```python
from build123d import *

# Parameters (mm, degrees)
SKETCH1_R               = 2.5
SKETCH1_W               = 6.5
SKETCH1_H               = 5
BOSS_EXTRUDE1_DEPTH     = 3
SKETCH1_3_W             = 6.5
SKETCH1_3_H             = 5
BOSS_EXTRUDE2_DEPTH     = 5.5
BOSS_EXTRUDE3_START     = -3
SKETCH2_W               = 3
SKETCH2_H               = 24
SKETCH2_H_2             = 3
SKETCH2_W_2             = 13
BOSS_EXTRUDE3_DEPTH     = 46
CUT_EXTRUDE1_DEPTH      = 56.497747702
CUT_EXTRUDE1_DEPTH_BACK = 56.497747702
CUT_EXTRUDE2_START      = -1
SKETCH4_R               = 1.75
CUT_EXTRUDE2_DEPTH      = 57.201398584
SKETCH4_2_R             = 1.75
CUT_EXTRUDE3_DEPTH      = 58.201398584
FILLET1_R               = 0.7


with BuildPart() as part:
    # Sketch1 → Boss-Extrude1 (new body)
    # profile 1 of 3: a face of its own
    with BuildSketch(Plane(origin=(0, 0, 0), x_dir=(1, 0, 0), z_dir=(0, 1, 0))):
        Polygon((-8, 30), (-8, 0), (-3.25, 0), (-3.25, 5), (3.25, 5), (3.25, 0), (8, 0), (8, 30), (3.25, 30), (3.25, 25), (-3.25, 25), (-3.25, 30), align=None)
        with Locations(Location((0, 15, 0), (0, 0, 270))):
            Circle(SKETCH1_R, mode=Mode.SUBTRACT)
    # profile 2 of 3: a face of its own
    with BuildSketch(Plane(origin=(0, 0, 0), x_dir=(1, 0, 0), z_dir=(0, 1, 0))):
        with Locations((0, 2.5)):
            Rectangle(SKETCH1_W, SKETCH1_H)
    # profile 3 of 3: a face of its own
    with BuildSketch(Plane(origin=(0, 0, 0), x_dir=(1, 0, 0), z_dir=(0, 1, 0))):
        with Locations((0, 27.5)):
            Rectangle(SKETCH1_W, SKETCH1_H)
    extrude(amount=BOSS_EXTRUDE1_DEPTH)

    # Sketch1<3> → Boss-Extrude2 (add)
    with BuildSketch(Plane(origin=(0, 0, 0), x_dir=(1, 0, 0), z_dir=(0, 1, 0))):
        with Locations((0, 27.5)):
            Rectangle(SKETCH1_3_W, SKETCH1_3_H)
        with Locations((0, 2.5)):
            Rectangle(SKETCH1_3_W, SKETCH1_3_H)
    extrude(amount=-BOSS_EXTRUDE2_DEPTH)

    # Sketch2 → Boss-Extrude3 (add)
    with BuildSketch(Plane(origin=(0, 3, 0), x_dir=(1, 0, 0), z_dir=(0, 1, 0)).offset(BOSS_EXTRUDE3_START)):
        with Locations((-6.5, 15)):
            Rectangle(SKETCH2_W, SKETCH2_H)
        with Locations((-6.5, 1.5)):
            Rectangle(SKETCH2_W, SKETCH2_H_2)
        with Locations((-6.5, 28.5)):
            Rectangle(SKETCH2_W, SKETCH2_H_2)
        with Locations((1.5, 28.5)):
            Rectangle(SKETCH2_W_2, SKETCH2_H_2)
        with Locations((1.5, 1.5)):
            Rectangle(SKETCH2_W_2, SKETCH2_H_2)
    extrude(amount=BOSS_EXTRUDE3_DEPTH)

    # Sketch3 → Cut-Extrude1 (cut, two sides: drawn at the far end of the back side and taken through both)
    with BuildSketch(Plane(origin=(0, 0, -30), x_dir=(-1, 0, 0), z_dir=(0, 0, -1)).offset(-CUT_EXTRUDE1_DEPTH_BACK)):
        Polygon((-8, 6), (2, 46), (-8, 46), align=None)
    extrude(amount=CUT_EXTRUDE1_DEPTH + CUT_EXTRUDE1_DEPTH_BACK, mode=Mode.SUBTRACT)

    # Sketch4 → Cut-Extrude2 (cut, through all)
    # profile 1 of 2: a face of its own
    with BuildSketch(Plane.ZY.offset(8).offset(CUT_EXTRUDE2_START)):
        Polygon((-8.556624327, 29.5), (-7.113248654, 32), (-8.556624327, 34.5), (-11.443375673, 34.5), (-12.886751346, 32), (-11.443375673, 29.5), align=None)
        with Locations((-10, 32)):
            Circle(SKETCH4_R, mode=Mode.SUBTRACT)
    # profile 2 of 2: a face of its own
    with BuildSketch(Plane.ZY.offset(8).offset(CUT_EXTRUDE2_START)):
        Polygon((-18.556624327, 29.5), (-17.113248654, 32), (-18.556624327, 34.5), (-21.443375673, 34.5), (-22.886751346, 32), (-21.443375673, 29.5), align=None)
        with Locations((-20, 32)):
            Circle(SKETCH4_R, mode=Mode.SUBTRACT)
    extrude(amount=-CUT_EXTRUDE2_DEPTH, mode=Mode.SUBTRACT)

    # Sketch4<2> → Cut-Extrude3 (cut, through all)
    with BuildSketch(Plane.ZY.offset(8)):
        with Locations((-20, 32)):
            Circle(SKETCH4_2_R)
        with Locations((-10, 32)):
            Circle(SKETCH4_2_R)
    extrude(amount=-CUT_EXTRUDE3_DEPTH, mode=Mode.SUBTRACT)

    # Fillet1
    fillet1_edges = [part.edges().sort_by_distance(p)[0] for p in [
        (3, 26, -30),
        (3, 26, -27),
        (3, 26, 0),
        (3, 26, -3),
    ]]
    fillet(fillet1_edges, radius=FILLET1_R)


solid = part.part
```
CAD build for the part. Positions are in the model's coordinates, mm. A direction names the side the tool comes from. Give positions to 0.01 mm unless a question says otherwise; leave off trailing zeros. Loops run counter-clockwise (first coordinate to the right, second up) from the corner with the lowest first, then second, coordinate; pieces in that order, holes last. Notation, with made-up numbers: (-7.5, 76) - (29.5, 76) arc R19 cw to (29.5, 82) - close; hole circle Ø7 at (80, 64.5). An arc over 180 degrees is marked (long way). Put each result on its own line as item: value.
Q1. Mould opens along Y. For faces 4 (the face through (-6.014, 33.232, -7.825)), 5 (the face through (-5, 24, -15)), 6 (the face through (3.19, 24.38, -0.2)) say: pulls with the +Y half, pulls with the -Y half, needs draft (parallel to the pull), parting line crosses it, or undercut.
Filled in:
face 4: undercut
face 5: needs draft
face 6: pulls with the +Y half
Q2. Slice it at D-D (x = -3.75). Give the cut face in (y, z).
Filled in:
outline: (0, -30) - (46, -30) - (46, -27) - (3, -27) - (3, -3) - (46, -3) - (46, 0) - (0, 0) - close
Q3. Probe line 1 along Z through (x, y) = (3, 10.5); line 2 along X through (y, z) = (2.25, -15); line 3 along Y through (x, z) = (-7.25, -10). List the from-to ranges inside material, lowest first.
Filled in:
line 1: z = -30 to -27, -3 to 0
line 2: x = -8 to -2.5, 2.5 to 8
line 3: y = 0 to 30.25, 33.75 to 46
Q4. Slice it at B-B (x = -6.25). Give the cut face in (y, z).
Filled in:
outline: (0, -30) - (46, -30) - (46, 0) - (0, 0) - close; hole (29.5, -21.44) - (32, -22.89) - (34.5, -21.44) - (34.5, -18.56) - (32, -17.11) - (29.5, -18.56) - close; hole (29.5, -11.44) - (32, -12.89) - (34.5, -11.44) - (34.5, -8.56) - (32, -7.11) - (29.5, -8.56) - close
Q5. Slice it at C-C (z = -1.75). Give the cut face in (x, y), plus the area to 3 significant figures.
Filled in:
outline: (-8, 0) - (-3.25, 0) - (-3.25, -5.5) - (3.25, -5.5) - (3.25, 0) - (8, 0) - (8, 6) - (-2, 46) - (-8, 46) - close
area: 572 mm²
Q6. Flat gauge pins, fed straight in: pin 1 (1 mm diameter, centred on x = 3, z = -26, fed in from +Y); pin 2 (1.5 mm diameter, centred on y = -2, z = -28, fed in from +X); pin 3 (4 mm diameter, centred on y = 33, z = -10, fed in from +X). Where does each tip first touch, or does it go through?
Filled in:
pin 1: stops at y = 3
pin 2: stops at x = 3.25
pin 3: stops at x = -5
Q7. Slice it at A-A (z = -10). Give the cut face in (x, y), plus the area to 4 significant figures.
Filled in:
outline: (-8, 0) - (8, 0) - (8, 3) - (-5, 3) - (-5, 29.5) - (-7, 29.5) - (-7, 30.25) - (-8, 30.25) - close; (-8, 33.75) - (-7, 33.75) - (-7, 34.5) - (-5, 34.5) - (-5, 46) - (-8, 46) - close
area: 163.5 mm²
Q8. Tool access for faces 1 (the face through (3, 3, -15)), 2 (the face through (-7, 34, -9)), 3 (the face through (0, -3, -5)): list every direction of +Z, -Z, +X, -X, +Y, -Y with a clear straight run to the whole face (end or side of a thin tool).
Filled in:
face 1: +X, +Y
face 2: +X
face 3: +X, -X, -Y
